For this review, take the finished solid that the model builds, in its own axes (mm). Face numbers are marked on the shaded views. Coordinates: 2 decimals unless noted, no trailing zeros.
from build123d import *

# Parameters (mm, degrees)
PAD_DEPTH       = 4
POCKET_DEPTH    = 4.4
SKETCH003_R     = 1.3
POCKET001_DEPTH = 60.935119
SKETCH004_R     = 2.5
POCKET002_DEPTH = 57.935119
FILLET_R        = 0.89


with BuildPart() as part:
    # Sketch001 → Pad (new body, symmetric)
    with BuildSketch(Plane.XY):
        Polygon((-63.75, 0), (-26.029329, 65.334119), (63.75, 13.5), (63.75, 0), (50.75, 0), (50.75, 5.5), (-36.25, 5.5), (-36.25, 0), align=None)
        Polygon((-49.027568, 13.5), (-23.833176, 57.137967), (51.75, 13.5), align=None, mode=Mode.SUBTRACT)
    extrude(amount=PAD_DEPTH, both=True)

    # Sketch002 → Pocket (cut)
    with BuildSketch(Plane.XZ):
        with BuildLine():
            ThreePointArc((-56.25, -3.1), (-53.15, 0), (-56.25, 3.1))
            Line((-56.25, 3.1), (-56.25, 4))
            Line((-56.25, 4), (-63.75, 4))
            Line((-63.75, 4), (-63.75, -4))
            Line((-63.75, -4), (-56.25, -4))
            Line((-56.25, -3.1), (-56.25, -4))
        make_face()
        with BuildLine():
            ThreePointArc((58.75, 3.1), (55.65, 0), (58.75, -3.1))
            Line((58.75, -3.1), (58.75, -4))
            Line((63.75, -4), (58.75, -4))
            Line((63.75, 4), (63.75, -4))
            Line((58.75, 4), (63.75, 4))
            Line((58.75, 3.1), (58.75, 4))
        make_face()
    extrude(amount=-POCKET_DEPTH, mode=Mode.SUBTRACT)

    # Sketch003 → Pocket001 (cut, through all)
    with BuildSketch(Plane.XZ.offset(-4.4)):
        with Locations((-56.25, 0)):
            Circle(SKETCH003_R)
        with Locations((58.75, 0)):
            Circle(SKETCH003_R)
    extrude(amount=-POCKET001_DEPTH, mode=Mode.SUBTRACT)

    # Sketch004 → Pocket002 (cut, through all)
    with BuildSketch(Plane.XZ.offset(-7.4)):
        with Locations((-56.25, 0)):
            Circle(SKETCH004_R)
        with Locations((58.75, 0)):
            Circle(SKETCH004_R)
    extrude(amount=-POCKET002_DEPTH, mode=Mode.SUBTRACT)

    # Fillet
    fillet_edges = [part.edges().sort_by_distance(p)[0] for p in [
        (-43.619494, 34.86706, -4),
        (18.860336, 39.41706, -4),
        (63.75, 8.95, -4),
        (61.25, 4.4, -4),
        (58.75, 2.2, -4),
        (54.75, 0, -4),
        (50.75, 2.75, -4),
        (7.25, 5.5, -4),
        (-36.25, 2.75, -4),
        (-46.25, 0, -4),
        (-56.25, 2.2, -4),
        (-58.729829, 4.4, -4),
        (-36.430372, 35.318984, -4),
        (1.361216, 13.5, -4),
        (13.958412, 35.318984, -4),
        (-43.619494, 34.86706, 4),
        (18.860336, 39.41706, 4),
        (63.75, 8.95, 4),
        (61.25, 4.4, 4),
        (58.75, 2.2, 4),
        (54.75, 0, 4),
        (50.75, 2.75, 4),
        (7.25, 5.5, 4),
        (-36.25, 2.75, 4),
        (-46.25, 0, 4),
        (-56.25, 2.2, 4),
        (-58.729829, 4.4, 4),
        (-36.430372, 35.318984, 4),
        (1.361216, 13.5, 4),
        (13.958412, 35.318984, 4),
        (63.75, 4.4, 0),
        (63.75, 13.5, 0),
        (-49.027568, 13.5, 0),
        (-23.833176, 57.137967, 0),
        (51.75, 13.5, 0),
        (-26.029329, 65.334119, 0),
        (-61.209659, 4.4, 0),
        (-56.25, 0, 3.55),
        (-56.25, 0, -3.55),
        (-36.25, 0, 0),
        (50.75, 0, 0),
    ]]
    fillet(fillet_edges, radius=FILLET_R)


solid = part.part
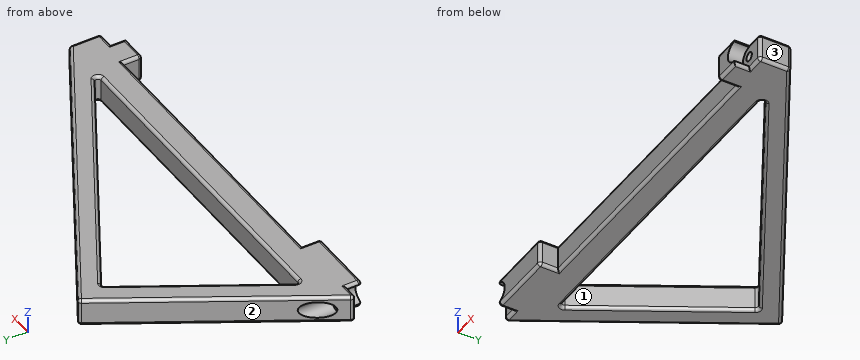
1. Take a section at A-A, the plane z = 0. Give the number of separate pieces and of enclosed holes in the cut face, plus the area to 3 significant figures.
Answer below:
separate pieces: 3
enclosed holes: 1
area: 1,930 mm2
2. The part is to be moulded in two halves that separate along Y. For the marked faces 1, 2 and 3, say which applies: +Y half, -Y half, draft (parallel to the pull), parting line (faces both ways), or undercut.
Answer below:
face 1: undercut
face 2: +Y half
face 3: draft
3. Clearance check with flat-ended pins moving along their axes: pin 1 Ø1.5 at (x, z) = (27, 1.5) entering from -Y; pin 2 Ø4 at (x, z) = (8.5, 0.5) entering from +Y; pin 3 Ø3.5 at (x, z) = (58.75, 0) entering from +Y. State where each tip first meets the part, or that it passes through.
Answer below:
pin 1: stops at y = 5.5
pin 2: stops at y = 46.55
pin 3: stops at y = 7.4
4. To check wall thickness, follow L1, parallel to Z at x = -56.25, y = 5.1; L2, parallel to X at y = 14, z = -0.25; L3, parallel to X at y = 7, z = -0.5. State the ranges of each line that lie inside material, in increasing order.
Answer below:
L1: z = -3.98 to -1.3, 1.3 to 3.98
L2: x = -53.76 to -48.29, 49.23 to 56.26, 61.24 to 62.88
L3: x = -59.71 to -57.45, -55.05 to 57.55, 59.95 to 63.75
